Part print with two shaded views. Sizes in mm from the minimum x, y, z corner. A direction names the side the tool comes from. Round coordinates to 2 decimals unless told otherwise and drop trailing zeros. Order: outer loops, then holes, each group sorted by start corner. A loop starts at its lowest first (then second) coordinate and runs counter-clockwise, first axis right, second up. Notation, with made-up numbers: (14.25, 88.25) - (52.25, 88.25) arc R17 cw to (52.25, 112.25) - close; hole circle Ø9 at (59, 68). An arc over 180 degrees is marked (long way). Write item = value, one per line.
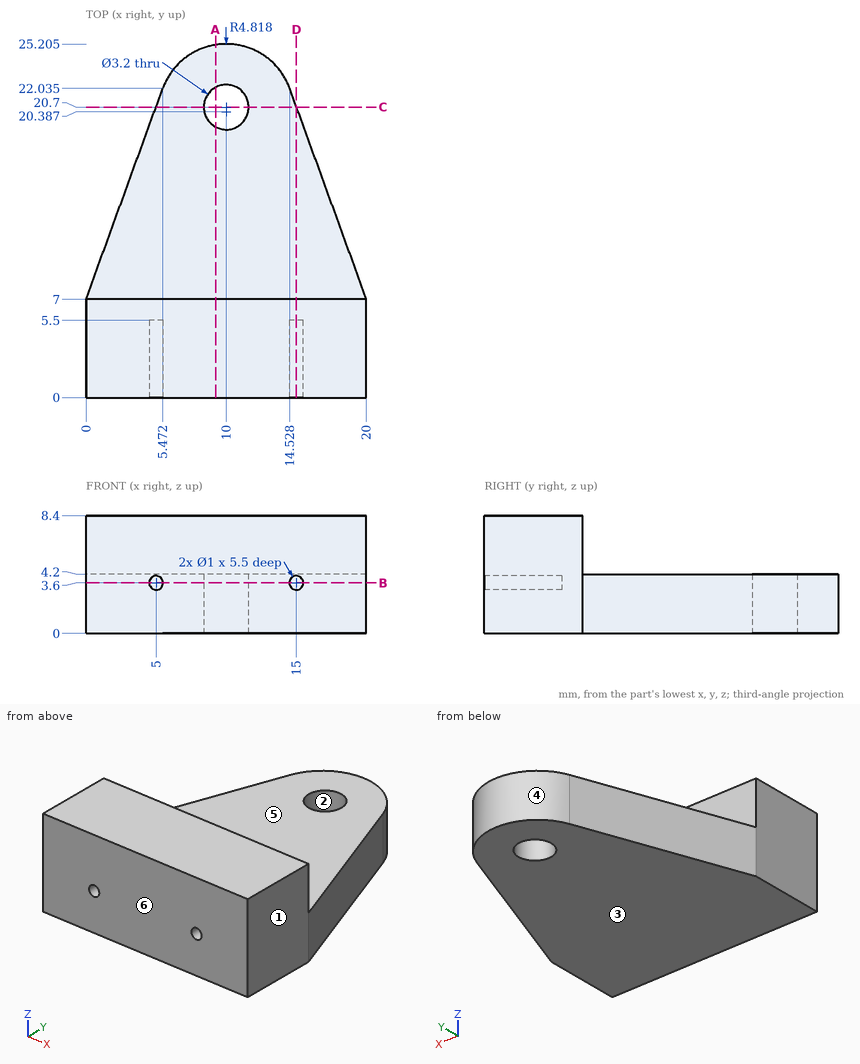
1) Cut at C-C (y = 20.7). Write the cut outline in (x, z).
Conclusion:
outline = (4.99, 0) - (8.4, 0) - (8.4, 4.2) - (4.99, 4.2) - close; (11.6, 0) - (15.01, 0) - (15.01, 4.2) - (11.6, 4.2) - close
2) Mould opens along X. For the marked faces 1, 2, 3 and 4 say: +X half, -X half, draft (parallel to the pull), parting line (faces both ways), or undercut.
Conclusion:
face_1 = +X half
face_2 = undercut
face_3 = draft
face_4 = parting line
3) Wall check: line 1 along Z through (x, y) = (5, 3.05); line 2 along Y through (x, z) = (10, 2.9) (1 decimal); line 3 along X through (y, z) = (19.75, 2). Give the ranges that are in metal, low to high.
Conclusion:
line_1 = 0 to 3.1, 4.1 to 8.4
line_2 = 0 to 19.1, 22.3 to 25.2
line_3 = 4.64 to 8.71, 11.29 to 15.36
4) Flat gauge pins, fed straight in: pin 1 Ø4 at (y, z) = (18.5, 1.5) entering from -X; pin 2 Ø1 at (y, z) = (16.5, 1.5) entering from -X (1 decimal); pin 3 Ø2.5 at (x, y) = (10, 20.7) entering from -Z; pin 4 Ø4 at (x, y) = (15, 18.5) entering from +Z. Where does each tip first touch, or does it go through?
Conclusion:
pin_1 = 3.46
pin_2 = 3.3
pin_3 = through
pin_4 = 4.2
5) Cut at B-B (z = 3.6). Write the cut outline in (x, y) (1 decimal), and give its area (3 significant figures).
Conclusion:
outline = (0, 0) - (4.5, 0) - (4.5, 5.5) - (5.5, 5.5) - (5.5, 0) - (14.5, 0) - (14.5, 5.5) - (15.5, 5.5) - (15.5, 0) - (20, 0) - (20, 7) - (14.5, 22) arc R4.8 ccw to (5.5, 22) - (0, 7) - close; hole circle Ø3.2 at (10, 20.7)
area = 360 mm^2
6) Cut at D-D (x = 15). Write the cut outline in (y, z).
Conclusion:
outline = (0, 0) - (20.74, 0) - (20.74, 4.2) - (7, 4.2) - (7, 8.4) - (0, 8.4) - (0, 4.1) - (5.5, 4.1) - (5.5, 3.1) - (0, 3.1) - close
7) Cut at A-A (x = 9.25). Write the cut outline in (y, z), and give its area (3 significant figures).
Conclusion:
outline = (0, 0) - (19.29, 0) - (19.29, 4.2) - (7, 4.2) - (7, 8.4) - (0, 8.4) - close; (22.11, 0) - (25.15, 0) - (25.15, 4.2) - (22.11, 4.2) - close
area = 123 mm^2
8) 3-axis set-ups, long thin cutter, end or side, ignore diameter. For the marked faces 5 and 6: which of +Z, -Z, +X, -X, +Y, -Y reach the whole face in a straight line?
Conclusion:
face_5 = +Z, +X, -X, +Y
face_6 = +Z, -Z, +X, -X, -Y
